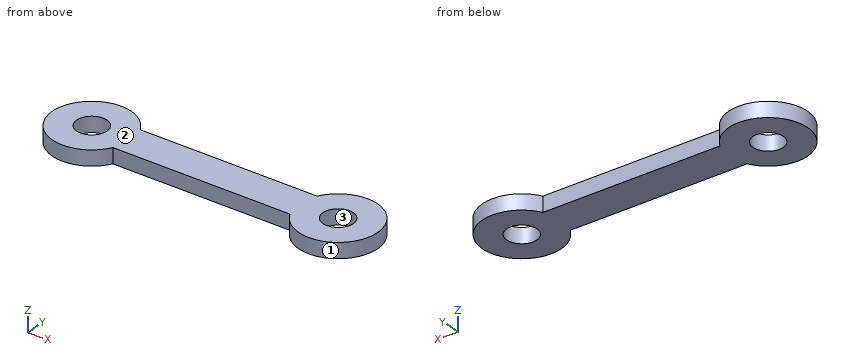
```python
from build123d import *

# Parameters (mm, degrees)
SKETCH_R  = 2.5
PAD_DEPTH = 2.5


with BuildPart() as part:
    # Sketch → Pad (new body)
    with BuildSketch(Plane.XY):
        with BuildLine():
            Line((-14.75, 3), (14.75, 3))
            ThreePointArc((14.75, -3), (27.016281, 0), (14.75, 3))
            Line((14.75, -3), (-14.75, -3))
            ThreePointArc((-14.75, 3), (-27.016281, 0), (-14.75, -3))
        make_face()
        with Locations((-20.516281, 0)):
            Circle(SKETCH_R, mode=Mode.SUBTRACT)
        with Locations((20.516281, 0)):
            Circle(SKETCH_R, mode=Mode.SUBTRACT)
    extrude(amount=PAD_DEPTH)


solid = part.part
```
Model file for the job. Use its own axes, mm. Face numbers are marked on the shaded views. Coordinates: 2 decimals unless noted, no trailing zeros. Loops run counter-clockwise (first coordinate to the right, second up) from the corner with the lowest first, then second, coordinate; pieces in that order, holes last. Notation, with made-up numbers: (-10.75, 44) - (12.25, 44) arc R8 ccw to (12.25, 50) - close; hole circle Ø3 at (-13, -36). An arc over 180 degrees is marked (long way). Write item = value, one per line. Start each with the question number.
Item 1: Saw through at C-C, the plane x = 20.5. List the corners of the cut face in (y, z), then the cut area to 3 significant figures.
Item 2: Saw through at B-B, the plane z = 1.9. List the corners of the cut face in (x, y).
Item 3: Pull direction Y, two halves, no side cores. Call the marked faces 1, 2 and 3: +Y half, -Y half, draft (parallel to the pull), parting line (faces both ways), or undercut.
Item 4: Saw through at A-A, the plane y = 0. List the corners of the cut face in (x, z).
Item 5: Wall check: probe 1 along X at (y, z) = (0.75, 2.1); probe 2 along X at (y, z) = (-0.5, 1.4); probe 3 along X at (y, z) = (6, 2.05). Give the ranges that are in metal, low to high. Write a range as [from, to].
Item 6: Saw through at D-D, the plane y = -4.25. List the corners of the cut face in (x, z).
Item 7: Drop a flat-ended pin along its axis: pin 1 Ø0.8 at (x, z) = (-5, 1.5) entering from -Y. Give the stop position or say it passes through.
Answers:
q1.outline = (-6.5, 0) - (-2.5, 0) - (-2.5, 2.5) - (-6.5, 2.5) - close; (2.5, 0) - (6.5, 0) - (6.5, 2.5) - (2.5, 2.5) - close
q1.area = 20.0 mm2
q2.outline = (-14.75, -3) - (14.75, -3) arc R6.5 ccw (long way) to (14.75, 3) - (-14.75, 3) arc R6.5 ccw (long way) to start; hole circle Ø5 at (-20.52, 0); hole circle Ø5 at (20.52, 0)
q3.face_1 = parting line
q3.face_2 = draft
q3.face_3 = undercut
q4.outline = (-27.02, 0) - (-23.02, 0) - (-23.02, 2.5) - (-27.02, 2.5) - close; (-18.02, 0) - (18.02, 0) - (18.02, 2.5) - (-18.02, 2.5) - close; (23.02, 0) - (27.02, 0) - (27.02, 2.5) - (23.02, 2.5) - close
q5.probe_1 = [-26.97, -22.9], [-18.13, 18.13], [22.9, 26.97]
q5.probe_2 = [-27, -22.97], [-18.07, 18.07], [22.97, 27]
q5.probe_3 = [-23.02, -18.02], [18.02, 23.02]
q6.outline = (-25.43, 0) - (-15.6, 0) - (-15.6, 2.5) - (-25.43, 2.5) - close; (15.6, 0) - (25.43, 0) - (25.43, 2.5) - (15.6, 2.5) - close
q7.pin_1 = -3
